from build123d import *

# Parameters (mm, degrees)
SKETCH1_W           = 40
SKETCH1_H           = 80
BOSS_EXTRUDE1_DEPTH = 5
SKETCH2_R           = 11
CUT_EXTRUDE1_DEPTH  = 5
SKETCH3_R           = 1.5
CUT_EXTRUDE2_DEPTH  = 5
SKETCH4_R           = 1.5
CUT_EXTRUDE3_DEPTH  = 5
SKETCH6_R           = 19
CUT_EXTRUDE4_DEPTH  = 1.7
SKETCH7_R           = 7
CUT_EXTRUDE5_DEPTH  = 45.842948164
CUT_EXTRUDE6_DEPTH  = 46
BOSS_EXTRUDE2_DEPTH = 5
BOSS_EXTRUDE3_START = 10
BOSS_EXTRUDE3_DEPTH = 10
BOSS_EXTRUDE4_DEPTH = 15
SKETCH12_R          = 3
CUT_EXTRUDE7_DEPTH  = 15
SKETCH13_R          = 4
CUT_EXTRUDE8_DEPTH  = 15


with BuildPart() as part:
    # Sketch1 → Boss-Extrude1 (new body)
    with BuildSketch(Plane.XY):
        Rectangle(SKETCH1_W, SKETCH1_H)
    extrude(amount=BOSS_EXTRUDE1_DEPTH)

    # Sketch2 → Cut-Extrude1 (cut)
    with BuildSketch(Plane.XY.offset(5)):
        with Locations((0, 20)):
            Circle(SKETCH2_R)
    extrude(amount=-CUT_EXTRUDE1_DEPTH, mode=Mode.SUBTRACT)

    # Sketch3 → Cut-Extrude2 (cut)
    with BuildSketch(Plane(origin=(0, 0, 0), x_dir=(-1, 0, 0), z_dir=(0, 0, -1))):
        with Locations((0, 34.9)):
            Circle(SKETCH3_R)
        with Locations((12.903778516, 12.55)):
            Circle(SKETCH3_R)
        with Locations((-12.903778516, 12.55)):
            Circle(SKETCH3_R)
    extrude(amount=-CUT_EXTRUDE2_DEPTH, mode=Mode.SUBTRACT)

    # Sketch4 → Cut-Extrude3 (cut)
    with BuildSketch(Plane(origin=(0, 0, 0), x_dir=(-1, 0, 0), z_dir=(0, 0, -1))):
        with Locations((0, -7.5)):
            Circle(SKETCH4_R)
        with Locations((0, -32.5)):
            Circle(SKETCH4_R)
    extrude(amount=-CUT_EXTRUDE3_DEPTH, mode=Mode.SUBTRACT)

    # Sketch6 → Cut-Extrude4 (cut)
    with BuildSketch(Plane(origin=(0, 0, 0), x_dir=(-1, 0, 0), z_dir=(0, 0, -1))):
        with Locations((0, -20)):
            Circle(SKETCH6_R)
    extrude(amount=-CUT_EXTRUDE4_DEPTH, mode=Mode.SUBTRACT)

    # Sketch7 → Cut-Extrude5 (cut, through all)
    with BuildSketch(Plane(origin=(0, 0, 1.7), x_dir=(-1, 0, 0), z_dir=(0, 0, -1))):
        with Locations((0, -20)):
            Circle(SKETCH7_R)
    extrude(amount=-CUT_EXTRUDE5_DEPTH, mode=Mode.SUBTRACT)

    # Sketch8 → Cut-Extrude6 (cut, through all)
    with BuildSketch(Plane(origin=(0, 0, 0), x_dir=(-1, 0, 0), z_dir=(0, 0, -1))):
        with BuildLine():
            Line((-20, 40), (-20, 20))
            ThreePointArc((-20, 20), (-14.142135605, 34.142135642), (5.2e-08, 40))
            Line((5.2e-08, 40), (-20, 40))
        make_face()
        with BuildLine():
            Line((20, 40), (5.2e-08, 40))
            ThreePointArc((5.2e-08, 40), (14.142135642, 34.142135605), (20, 20))
            Line((20, 20), (20, 40))
        make_face()
        with BuildLine():
            ThreePointArc((-6e-09, -40), (-14.142135626, -34.142135622), (-20, -20))
            Line((-20, -20), (-20, -40))
            Line((-20, -40), (-6e-09, -40))
        make_face()
        with BuildLine():
            ThreePointArc((20, -20), (14.142135622, -34.142135626), (-6e-09, -40))
            Line((-6e-09, -40), (20, -40))
            Line((20, -40), (20, -20))
        make_face()
    extrude(amount=-CUT_EXTRUDE6_DEPTH, mode=Mode.SUBTRACT)

    # Sketch9 → Boss-Extrude2 (add)
    with BuildSketch(Plane(origin=(0, 0, 0), x_dir=(-1, 0, 0), z_dir=(0, 0, -1))):
        with BuildLine():
            Line((20, 20), (20, 5))
            ThreePointArc((20, 5), (0, 45), (-20, 5))
            Line((-20, 5), (-20, 20))
            ThreePointArc((-20, 20), (0, 40), (20, 20))
        make_face()
    extrude(amount=-BOSS_EXTRUDE2_DEPTH)

    # Sketch10 → Boss-Extrude3 (add)
    with BuildSketch(Plane(origin=(0, 0, 0), x_dir=(-1, 0, 0), z_dir=(0, 0, -1)).offset(BOSS_EXTRUDE3_START)):
        with BuildLine():
            Line((20, 20), (25, 20))
            ThreePointArc((25, 20), (0, 45), (-25, 20))
            Line((-25, 20), (-20, 20))
            ThreePointArc((-20, 20), (0, 40), (20, 20))
        make_face()
    extrude(amount=-BOSS_EXTRUDE3_DEPTH)

    # Sketch11 → Boss-Extrude4 (add)
    with BuildSketch(Plane(origin=(0, 0, -10), x_dir=(-1, 0, 0), z_dir=(0, 0, -1))):
        Polygon((-10, 42.912878475), (-7.5, 57.912878475), (8.5, 57.912878475), (10, 42.912878475), align=None)
    extrude(amount=-BOSS_EXTRUDE4_DEPTH)

    # Sketch12 → Cut-Extrude7 (cut)
    with BuildSketch(Plane(origin=(0, 57.912878475, 0), x_dir=(1, 0, 0), z_dir=(0, 1, 0))):
        with Locations(Location((-0.5, 2.5, 0), (0, 0, 270))):
            Circle(SKETCH12_R)
    extrude(amount=-CUT_EXTRUDE7_DEPTH, mode=Mode.SUBTRACT)

    # Sketch13 → Cut-Extrude8 (cut)
    with BuildSketch(Plane(origin=(0, 57.912878475, 0), x_dir=(1, 0, 0), z_dir=(0, 1, 0))):
        with Locations(Location((-0.5, 2.5, 0), (0, 0, 270))):
            Circle(SKETCH13_R)
    extrude(amount=-CUT_EXTRUDE8_DEPTH, mode=Mode.SUBTRACT)


solid = part.part
Check sheet for the modelled part. Datum: model origin and axes. Units: mm. A direction names the side the tool comes from. Coordinates: 2 decimals unless noted, no trailing zeros. Loops run counter-clockwise (first coordinate to the right, second up) from the corner with the lowest first, then second, coordinate; pieces in that order, holes last. Notation, with made-up numbers: (21.5, -1.5) -> (28.5, -1.5) arc R36 cw to (28.5, 35.5) -> close; hole circle Ø10 at (52.25, 71). An arc over 180 degrees is marked (long way). Answer in a Markdown table with one row per item.
1. Material ranges on line 1 along X through (y, z) = (35, 3); line 2 along Y through (x, z) = (4, 0.75); line 3 along Z through (x, y) = (-7.5, -31), recorded low to high. Write a range as [from, to].
Check values:
| item | result |
|---|---|
| line 1 | x = [-20, -1.5], [1.5, 20] |
| line 2 | y = [-39.6, -38.57], [-1.43, 9.75], [30.25, 57.91] |
| line 3 | z = [1.7, 5] |
2. Access from +Z, -Z, +X, -X, +Y, -Y to the whole of each face (thin tool, end or side, straight path). Record for faces 1 (the face through (6, 9, 0)), 2 (the face through (0, 42.913, -3)), 3 (the face through (20, -8, 2)).
Check values:
| item | result |
|---|---|
| face 1 | -Z, -Y |
| face 2 | +Y |
| face 3 | +Z, -Z, +X, -Y |
3. Sectioned sample at C-C, the plane x = -6. Record the boundary of the cut face in (y, z).
Check values:
| item | result |
|---|---|
| outline | (-39.08, 0) -> (-38.03, 0) -> (-38.03, 1.7) -> (-23.61, 1.7) -> (-23.61, 5) -> (-39.08, 5) -> close; (-16.39, 1.7) -> (-1.97, 1.7) -> (-1.97, 0) -> (10.78, 0) -> (10.78, 5) -> (-16.39, 5) -> close; (29.22, 0) -> (39.08, 0) -> (39.08, -10) -> (57.91, -10) -> (57.91, 5) -> (29.22, 5) -> close |
4. Release check for a two-part mould opening along Y. For faces 4 (the face through (-20, -8, 2)), 5 (the face through (-2.38, 9.26, 2.54)), 6 (the face through (-22, 20, -5)), 7 (the face through (12.21, 11.22, 2.46)) record: released by +Y, released by -Y, zero draft, split by the parting line, or undercut.
Check values:
| item | result |
|---|---|
| face 4 | zero draft |
| face 5 | undercut |
| face 6 | released by -Y |
| face 7 | undercut |
5. Sectioned sample at D-D, the plane y = 12.55. Record the boundary of the cut face in (x, z), then the cut area to 3 significant figures.
Check values:
| item | result |
|---|---|
| outline | (-23.86, 0) -> (-14.4, 0) -> (-14.4, 5) -> (-23.86, 5) -> close; (-11.4, 0) -> (-8.09, 0) -> (-8.09, 5) -> (-11.4, 5) -> close; (8.09, 0) -> (11.4, 0) -> (11.4, 5) -> (8.09, 5) -> close; (14.4, 0) -> (23.86, 0) -> (23.86, 5) -> (14.4, 5) -> close |
| area | 128 mm2 |
6. Go/stop test with flat-tipped pins: pin 1 (19 mm diameter, centred on x = 8.5, y = -20, fed in from -Z); pin 2 (2 mm diameter, centred on y = 0.5, z = -2.5, fed in from -X); pin 3 (8 mm diameter, centred on y = 6, z = 3, fed in from +X); pin 4 (5.5 mm diameter, centred on x = 22, z = -5, fed in from -Y). Record where each tip stops, or that it passes through.
Check values:
| item | result |
|---|---|
| pin 1 | stops at z = 1.7 |
| pin 2 | passes through |
| pin 3 | stops at x = 22.91 |
| pin 4 | stops at y = 20 |
7. Sectioned sample at B-B, the plane z = -2.5. Record the boundary of the cut face in (x, y), then the cut area to 3 significant figures.
Check values:
| item | result |
|---|---|
| outline | (-25, 20) -> (-20, 20) arc R20 cw to (20, 20) -> (25, 20) arc R25 ccw to (10, 42.91) -> (7.5, 57.91) -> (3.5, 57.91) -> (3.5, 42.91) -> (-4.5, 42.91) -> (-4.5, 57.91) -> (-8.5, 57.91) -> (-10, 42.91) arc R25 ccw to start |
| area | 475 mm2 |
8. Sectioned sample at A-A, the plane y = 34.9. Record the boundary of the cut face in (x, z).
Check values:
| item | result |
|---|---|
| outline | (-20.07, -10) -> (-13.34, -10) -> (-13.34, 0) -> (-1.5, 0) -> (-1.5, 5) -> (-20.07, 5) -> close; (1.5, 0) -> (13.34, 0) -> (13.34, -10) -> (20.07, -10) -> (20.07, 5) -> (1.5, 5) -> close |
